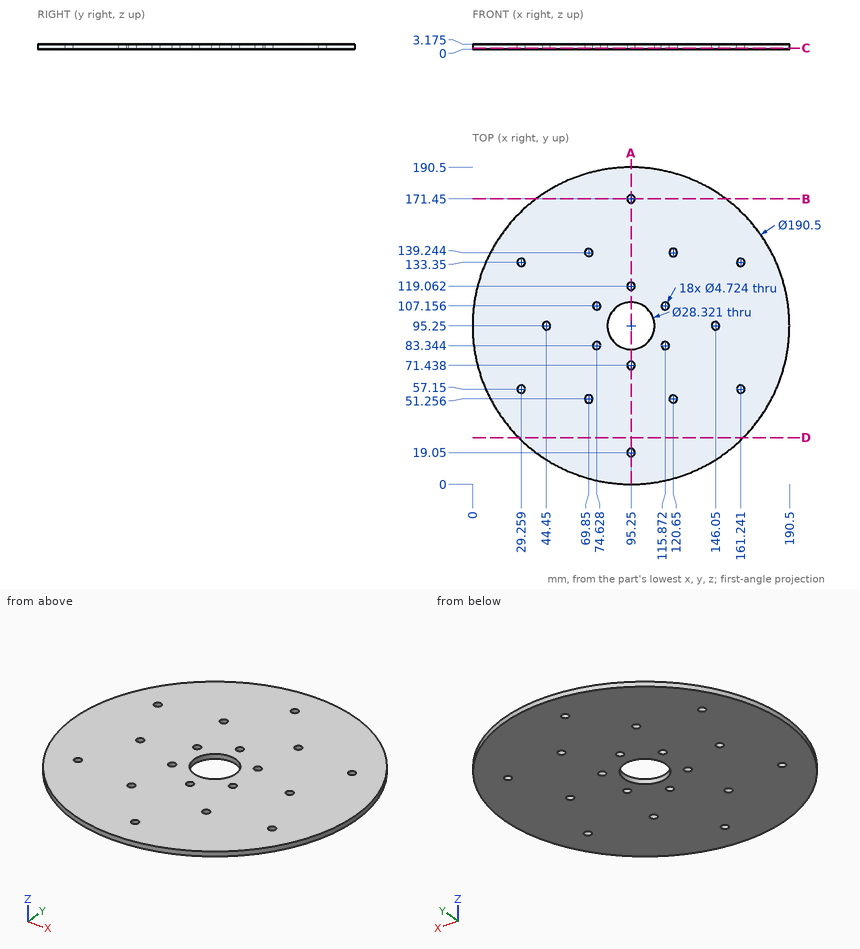
The figure shows three views and two pictorial views of one solid part (mm, origin at its lowest corner). Answer the questions. Give positions to 0.01 mm unless a question says otherwise; leave off trailing zeros. Write each loop counter-clockwise with the first axis right and the second up, starting at its lowest first coordinate (ties: lowest second). Pieces come first, ordered by that corner, then holes. Notation, with made-up numbers: (-5, 52.25) - (1, 52.25) arc R9 cw to (1, 68.25) - close; hole circle Ø9 at (24, 30.25). An arc over 180 degrees is marked (long way). Use CSV: the item, a comma, the result in double quotes. Start each with the question number.
Item 1: Consider line 1 (Y direction, x = 95.25, z = 1.1) (1 decimal); line 2 (Y direction, x = 30, z = 2.25) (1 decimal); line 3 (X direction, y = 59, z = 0.4) (1 decimal). Determine where each line is inside the solid, lowest interval first.
Item 2: The part is cut by section A-A, the plane x = 95.25. Give the vertices of the cut face in (y, z) (1 decimal).
Item 3: The part is cut by section C-C, the plane z = 0.7. Count the separate pieces of the cut face and the enclosed holes in it, and give its area (3 significant figures).
Item 4: The part is cut by section D-D, the plane y = 28. Give the vertices of the cut face in (x, z) (1 decimal).
Item 5: The part is cut by section B-B, the plane y = 171.45. Give the vertices of the cut face in (x, z) (1 decimal), and give its area (3 significant figures).
Item 6: Flat-ended cylindrical pins translate along their axes: P1, Ø3, axis at x = 95.25, y = 71.44, coming from the -Z side; P2, Ø1, axis at y = 75.5, z = 2.5, coming from the +X side (1 decimal). Find the tip coordinate at first contact, or state that the pin passes through.
Taken from the geometry:
1,line 1,"0 to 16.7, 21.4 to 69.1, 73.8 to 81.1, 109.4 to 116.7, 121.4 to 169.1, 173.8 to 190.5"
1,line 2,"25.9 to 54.9, 59.4 to 131.1, 135.6 to 164.6"
1,line 3,"7.2 to 27.8, 30.7 to 159.8, 162.7 to 183.3"
2,outline,"(0, 0) - (16.7, 0) - (16.7, 3.2) - (0, 3.2) - close; (21.4, 0) - (69.1, 0) - (69.1, 3.2) - (21.4, 3.2) - close; (73.8, 0) - (81.1, 0) - (81.1, 3.2) - (73.8, 3.2) - close; (109.4, 0) - (116.7, 0) - (116.7, 3.2) - (109.4, 3.2) - close; (121.4, 0) - (169.1, 0) - (169.1, 3.2) - (121.4, 3.2) - close; (173.8, 0) - (190.5, 0) - (190.5, 3.2) - (173.8, 3.2) - close"
3,separate pieces,"1"
3,enclosed holes,"19"
3,area,"27,600 mm2"
4,outline,"(27.8, 0) - (162.7, 0) - (162.7, 3.2) - (27.8, 3.2) - close"
5,outline,"(38.1, 0) - (92.9, 0) - (92.9, 3.2) - (38.1, 3.2) - close; (97.6, 0) - (152.4, 0) - (152.4, 3.2) - (97.6, 3.2) - close"
5,area,"348 mm2"
6,P1,"through"
6,P2,"x = 188.5"
